Study the drawing (mm; zero at the part's minimum x, y, z) and answer. Give positions to 0.01 mm unless a question says otherwise; leave off trailing zeros. Order: outer loops, then holes, each group sorted by start corner. A loop starts at its lowest first (then second) coordinate and runs counter-clockwise, first axis right, second up.
Item 1: A cutting plane is placed at B-B (x = 11.25). Write down the section's boundary in (y, z) (1 decimal), plus the area to 3 significant figures.
Item 2: A cutting plane is placed at C-C (x = 1.5). Write down the section's boundary in (y, z) (1 decimal).
Item 3: Given pin 1 Ø3 at (x, y) = (6.35, 7.33) entering from +Z; pin 2 Ø1.5 at (x, y) = (5.5, 8) entering from -Z (1 decimal), each flat-ended and moving along its own axis, determine where each tip first touches the part or whether it passes through.
Item 4: Find the intervals of material crossed by line 1 along Y through (x, z) = (6.35, 77.25) (1 decimal); line 2 along X through (y, z) = (9.5, 10) (1 decimal); line 3 along X through (y, z) = (5.5, 84.5) (1 decimal), in increasing order.
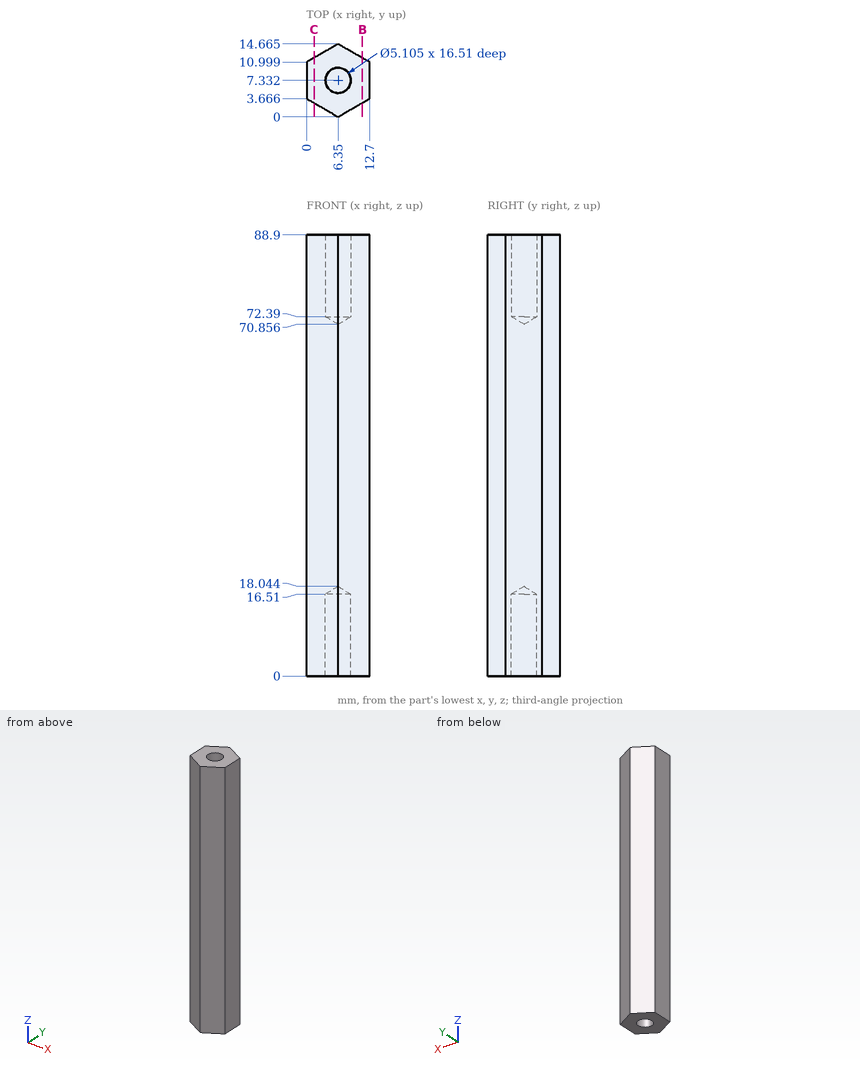
Response values:
1. outline: (2.8, 0) - (11.8, 0) - (11.8, 88.9) - (2.8, 88.9) - close
1. area: 801 mm2
2. outline: (2.8, 0) - (11.9, 0) - (11.9, 88.9) - (2.8, 88.9) - close
3. pin 1: stops at z = 71.76
3. pin 2: stops at z = 16.9
4. line 1: y = 0 to 4.8, 9.9 to 14.7
4. line 2: x = 0 to 5, 7.7 to 12.7
4. line 3: x = 0 to 4.6, 8.1 to 12.7
